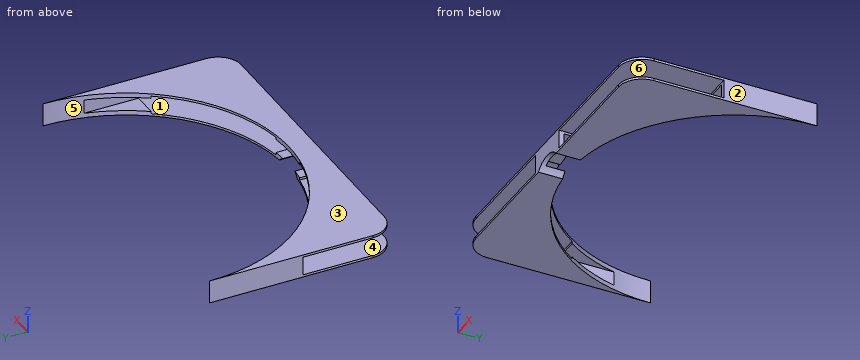
from build123d import *

# Parameters (mm, degrees)
F0_W     = 177.8
F0_H     = 12.7
F1_DEPTH = 101.6
F2_R     = 88.9
F3_DEPTH = 25.4
F4_T     = -2.54
F5_W     = 76.2
F5_H     = 10.16
F6_DEPTH = 50.8
F7_R     = 12.7
F8_R     = 12.7
F9_DEPTH = 25.4


with BuildPart() as f1:
    # F0 (on Front) → F1 (new body)
    with BuildSketch(Plane.XZ):
        with Locations((88.9, 6.35)):
            Rectangle(F0_W, F0_H)
    extrude(amount=-F1_DEPTH)

    # F2 (on face) → F3 (cut)
    with BuildSketch(Plane.XY.offset(12.7)):
        with Locations((88.9, 101.6)):
            Circle(F2_R)
    extrude(amount=-F3_DEPTH, mode=Mode.SUBTRACT)

    # F4
    f4_openings = [f1.faces().sort_by_distance(p)[0] for p in [
        (88.9, 12.7, 6.35),
    ]]
    offset(amount=F4_T, openings=f4_openings, kind=Kind.INTERSECTION)

    # F5 (on face) → F6 (cut)
    with BuildSketch(Plane.XZ):
        with Locations((38.1, 6.35)):
            Rectangle(F5_W, F5_H)
        with Locations((139.7, 6.35)):
            Rectangle(F5_W, F5_H)
    extrude(amount=-F6_DEPTH, mode=Mode.SUBTRACT)

    # F7
    f7_edges = [f1.edges().sort_by_distance(p)[0] for p in [
        (177.8, 0, 12.065),
        (177.8, 0, 0.635),
        (0, 0, 12.065),
        (0, 0, 0.635),
    ]]
    fillet(f7_edges, radius=F7_R)

    # F8 (on face) → F9 (cut)
    with BuildSketch(Plane.XZ):
        with Locations((88.9, -8.4582)):
            Circle(F8_R)
    extrude(amount=-F9_DEPTH, mode=Mode.SUBTRACT)


solid = f1.part
Design review of the part built by this model. Coordinates are the model's own, in mm. Face numbers are marked on the shaded views. A direction names the side the tool comes from. Round coordinates to 2 decimals unless told otherwise and drop trailing zeros. Order: outer loops, then holes, each group sorted by start corner. A loop starts at its lowest first (then second) coordinate and runs counter-clockwise, first axis right, second up. Notation, with made-up numbers: M 16.25,24.25 L 33.25,24.25 A8 cw 33.25,36.25 Z; hole C 58,45.5 d11. An arc over 180 degrees is marked long. Answer as CSV lines item,"result". Start each with the question number.
1) Wall thickness on line 1 along Z through (x, y) = (36.5, 15); line 2 along X through (y, z) = (52, 4.5); line 3 along Y through (x, z) = (86.5, 7): over which ranges is each line inside the solid? List them lowest first. Write a range as [from, to].
2) Add section B-B (x = 159). Give the boundary of the cut face in (y, z).
3) Tool access review of the marked faces 4, 5 and 6: name each direction out of +Z, -Z, +X, -X, +Y, -Y from which nothing blocks a thin tool from reaching the whole face with its end or side.
4) Add section C-C (y = 93). Give the boundary of the cut face in (x, z).
5) For pin 1 Ø12 at (x, y) = (43.5, 38) entering from +Z; pin 2 Ø5 at (y, z) = (4, 8.5) entering from +X; pin 3 Ø3 at (x, z) = (98, 2) entering from +Y; pin 4 Ø1.5 at (x, z) = (94.5, 11.5) entering from +Y, all flat-tipped, find the tip position at first contact; note any pin that passes through.
6) The part is to be moulded in two halves that separate along Z. For the marked faces 1, 2 and 3, say which applies: +Z half, -Z half, draft (parallel to the pull), parting line (faces both ways), or undercut.
7) Add section A-A (z = 7.5). Give the boundary of the cut face in (x, y).
8) Add section D-D (x = 88.9). Give the boundary of the cut face in (y, z).
Resolved:
1,line 1,"[0, 1.27], [11.43, 12.7]"
1,line 2,"[0, 2.54], [175.26, 177.8]"
1,line 3,"[0, 2.54]"
2,outline,"M 0,0 L 46.93,0 L 46.93,1.27 L 0,1.27 Z; M 0,11.43 L 46.93,11.43 L 46.93,12.7 L 0,12.7 Z"
3,face 4,"-X, -Y"
3,face 5,"+Z, -Z, +Y"
3,face 6,"+X, -Y"
4,outline,"M 0,0 L 0.42,0 L 0.42,12.7 L 0,12.7 Z; M 177.38,0 L 177.8,0 L 177.8,12.7 L 177.38,12.7 Z"
5,pin 1,"through"
5,pin 2,"x = 101.6"
5,pin 3,"y = 13.33"
5,pin 4,"y = 12.93"
6,face 1,"undercut"
6,face 2,"draft"
6,face 3,"+Z half"
7,outline,"M 0,50.8 L 2.54,50.8 L 2.54,80.5 A88.9 cw 0,101.6 Z; M 76.2,0 L 101.6,0 L 101.6,2.54 L 76.2,2.54 Z; M 175.26,50.8 L 177.8,50.8 L 177.8,101.6 A88.9 cw 175.26,80.5 Z"
8,outline,"M 0,4.24 L 2.54,4.24 L 2.54,10.16 L 12.7,10.16 L 12.7,12.7 L 0,12.7 Z"
